```python
from build123d import *

# Parameters (mm, degrees)
F0_W     = 609.6
F0_H     = 711.2
F1_DEPTH = 6.35
F2_R     = 76.2
F3_DEPTH = 692.15
F4_W     = 254
F4_H     = 304.8
F4_R     = 76.2
F5_DEPTH = 6.35


with BuildPart() as f1:
    # F0 (on Top) → F1 (new body)
    with BuildSketch(Plane.XY):
        Rectangle(F0_W, F0_H)
    extrude(amount=F1_DEPTH)

    # F2 (on face) → F3 (join)
    with BuildSketch(Plane.XY.offset(6.35)):
        Circle(F2_R)
    extrude(amount=F3_DEPTH)

    # F4 (on face) → F5 (join)
    with BuildSketch(Plane.XY.offset(698.5)):
        Rectangle(F4_W, F4_H)
        Circle(F4_R, mode=Mode.SUBTRACT)
        Circle(F4_R)
    extrude(amount=F5_DEPTH)


solid = f1.part
```
Geometry check sheet. Reference: the model listing, model coordinates, mm. Give positions to 0.01 mm unless a question says otherwise; leave off trailing zeros. Loops run counter-clockwise (first coordinate to the right, second up) from the corner with the lowest first, then second, coordinate; pieces in that order, holes last. Notation, with made-up numbers: (84.25, 60.25) - (113.25, 60.25) arc R19 ccw to (113.25, 89.25) - close; hole circle Ø9 at (87.5, 53.25). An arc over 180 degrees is marked (long way). Use CSV: the item, a comma, the result in double quotes. Start each with the question number.
Q1. Release check for a two-part mould opening along Z. For faces 1 (the face through (-60.47, -46.367, 347.58)), 2 (the face through (-4, 5, 0)), 3 (the face through (-2, 2, 704.85)) record: +Z half, -Z half, draft (parallel to the pull), parting line (faces both ways), or undercut.
Q2. Section check C-C, the plane z = 571.5. Record the cut outline in (x, y).
Q3. Go/stop test with flat-tipped pins: pin 1 Ø1 at (x, y) = (-80.5, -217.5) entering from +Z; pin 2 Ø1.9 at (y, z) = (-48, 703) entering from +X; pin 3 Ø1.5 at (x, z) = (51, 589) entering from +Y. Record where each tip stops, or that it passes through.
Q4. Section check D-D, the plane x = 252. Record the cut outline in (y, z), and give its area (3 significant figures).
Q5. Scan lines: probe 1 along Z at (x, y) = (-175, -73.5); probe 2 along X at (y, z) = (-4.5, 198); probe 3 along Y at (x, z) = (33, 124). Record each from-to range of solid material in increasing order. Write a range as from..to.
Q6. Section check B-B, the plane x = 0. Record the cut outline in (y, z).
Q7. Section check A-A, the plane y = 0. Record the cut outline in (x, z), and give its area (3 significant figures).
Findings below:
1,face 1,"undercut"
1,face 2,"-Z half"
1,face 3,"+Z half"
2,outline,"circle Ø152.4 at (0, 0)"
3,pin 1,"stops at z = 6.35"
3,pin 2,"stops at x = 127"
3,pin 3,"stops at y = 57.28"
4,outline,"(-355.6, 0) - (355.6, 0) - (355.6, 6.35) - (-355.6, 6.35) - close"
4,area,"4,520 mm^2"
5,probe 1,"z = 0..6.35"
5,probe 2,"x = -76.07..76.07"
5,probe 3,"y = -68.68..68.68"
6,outline,"(-355.6, 0) - (355.6, 0) - (355.6, 6.35) - (76.2, 6.35) - (76.2, 698.5) - (152.4, 698.5) - (152.4, 704.85) - (-152.4, 704.85) - (-152.4, 698.5) - (-76.2, 698.5) - (-76.2, 6.35) - (-355.6, 6.35) - close"
7,outline,"(-304.8, 0) - (304.8, 0) - (304.8, 6.35) - (76.2, 6.35) - (76.2, 698.5) - (127, 698.5) - (127, 704.85) - (-127, 704.85) - (-127, 698.5) - (-76.2, 698.5) - (-76.2, 6.35) - (-304.8, 6.35) - close"
7,area,"111,000 mm^2"
